```python
from build123d import *

# Parameters (mm, degrees)
SKETCH1_W            = 150
SKETCH1_H            = 150
BOSS_EXTRUDE2_DEPTH  = 3
SKETCH7_R            = 3
BOSS_EXTRUDE3_DEPTH  = 13
SKETCH13_W           = 15.146104274
SKETCH13_H           = 8
BOSS_EXTRUDE4_DEPTH  = 55
SKETCH14_W           = 100
SKETCH14_H           = 100
BOSS_EXTRUDE5_DEPTH  = 3
SKETCH15_R           = 3.001760758
SKETCH15_R_2         = 3.00141088
SKETCH15_R_3         = 3.000339641
SKETCH15_R_4         = 2.9990493
BOSS_EXTRUDE22_DEPTH = 15
SKETCH20_R           = 3
BOSS_EXTRUDE8_DEPTH  = 22.7
SKETCH23_W           = 52.466562125
SKETCH23_H           = 3
SKETCH23_W_2         = 9
BOSS_EXTRUDE9_DEPTH  = 5
BOSS_EXTRUDE10_DEPTH = 52.47
BOSS_EXTRUDE11_START = -74
BOSS_EXTRUDE11_DEPTH = 9
SKETCH25_W           = 9.00183775
SKETCH25_H           = 11.837712984
BOSS_EXTRUDE12_DEPTH = 8
SKETCH26_W           = 9
SKETCH26_H           = 5
SKETCH26_W_2         = 52.466562125
BOSS_EXTRUDE13_DEPTH = 43
SKETCH27_R           = 1.4
SKETCH27_W           = 35.7
SKETCH27_H           = 2.6
SKETCH27_W_2         = 23
SKETCH27_H_2         = 33
BOSS_EXTRUDE14_DEPTH = 2.4
SKETCH29_W           = 21.53
SKETCH29_H           = 48.531461908
BOSS_EXTRUDE15_DEPTH = 3
BOSS_EXTRUDE16_DEPTH = 21.53
BOSS_EXTRUDE17_DEPTH = 9
BOSS_EXTRUDE18_START = -30.53
BOSS_EXTRUDE18_DEPTH = 52.47
CUT_EXTRUDE5_DEPTH   = 8
BOSS_EXTRUDE19_DEPTH = 21.53
SKETCH21_R           = 1.5
BOSS_EXTRUDE20_DEPTH = 3
SKETCH17_R           = 1.5
BOSS_EXTRUDE21_DEPTH = 3
SKETCH15_3_R         = 1.75230345
SKETCH15_3_R_2       = 1.749240596
SKETCH15_3_R_3       = 1.752045419
SKETCH15_3_R_4       = 1.747263247
BOSS_EXTRUDE23_DEPTH = 18
SKETCH27_3_R         = 1.4
BOSS_EXTRUDE24_DEPTH = 4.4


with BuildPart() as part:
    # Sketch1 → Boss-Extrude2 (new body)
    with BuildSketch(Plane.XY):
        with Locations((121.156017968, 146.961713176)):
            Rectangle(SKETCH1_W, SKETCH1_H)
    extrude(amount=BOSS_EXTRUDE2_DEPTH)

    # Sketch7 → Boss-Extrude3 (add)
    with BuildSketch(Plane.XY):
        with Locations(Location((100.23733205, 77.422228763, 0), (0, 0, 180))):
            Circle(SKETCH7_R)
        with Locations(Location((177.53733205, 77.422228763, 0), (0, 0, 180))):
            Circle(SKETCH7_R)
        with Locations(Location((177.53733205, 119.222228763, 0), (0, 0, 180))):
            Circle(SKETCH7_R)
        with Locations(Location((100.23733205, 119.222228763, 0), (0, 0, 180))):
            Circle(SKETCH7_R)
    extrude(amount=BOSS_EXTRUDE3_DEPTH)

    # Sketch13 → Boss-Extrude4 (add)
    with BuildSketch(Plane.XY.offset(3)):
        Polygon((196.156017968, 213.964413798), (196.156017968, 221.961713176), (99.253187126, 221.961713176), (99.253187126, 213.964413798), (107.253187126, 213.964413798), align=None)
        Polygon((107.253187126, 213.964413798), (99.253187126, 213.964413798), (99.253187126, 126.654100723), (107.253187126, 126.654100723), (107.253187126, 136.806372616), (107.253187126, 144.806372616), align=None)
        Polygon((196.156017968, 136.806372616), (196.156017968, 144.806372616), (107.253187126, 144.806372616), (107.253187126, 136.806372616), (181.009913694, 136.806372616), align=None)
        with Locations((188.582965831, 132.806372616)):
            Rectangle(SKETCH13_W, SKETCH13_H)
    extrude(amount=BOSS_EXTRUDE4_DEPTH)

    # Sketch14 → Boss-Extrude5 (add)
    with BuildSketch(Plane.XY.offset(58)):
        with Locations((146.156017968, 171.961713176)):
            Rectangle(SKETCH14_W, SKETCH14_H)
    extrude(amount=BOSS_EXTRUDE5_DEPTH)

    # Sketch15 → Boss-Extrude22 (add)
    with BuildSketch(Plane.XY.offset(61)):
        with Locations(Location((103.656017968, 214.961713176, 0), (0, 0, 180))):
            Circle(SKETCH15_R)
        with Locations(Location((103.656017968, 129.961713176, 0), (0, 0, 180))):
            Circle(SKETCH15_R_2)
        with Locations(Location((188.656017968, 129.961713176, 0), (0, 0, 180))):
            Circle(SKETCH15_R_3)
        with Locations(Location((188.656017968, 214.961713176, 0), (0, 0, 180))):
            Circle(SKETCH15_R_4)
    extrude(amount=BOSS_EXTRUDE22_DEPTH)

    # Sketch20 → Boss-Extrude8 (add)
    with BuildSketch(Plane.XY.offset(3)):
        with Locations(Location((92.052701123, 214.281671575, 0), (0, 0, 180))):
            Circle(SKETCH20_R)
        with Locations(Location((52.052701123, 214.281671575, 0), (0, 0, 180))):
            Circle(SKETCH20_R)
        with Locations(Location((52.052701123, 174.281671575, 0), (0, 0, 180))):
            Circle(SKETCH20_R)
        with Locations(Location((92.052701123, 174.281671575, 0), (0, 0, 180))):
            Circle(SKETCH20_R)
        with Locations(Location((92.005217403, 161.997286282, 0), (0, 0, 180))):
            Circle(SKETCH20_R)
        with Locations(Location((52.005217403, 161.997286282, 0), (0, 0, 180))):
            Circle(SKETCH20_R)
        with Locations(Location((92.005217403, 121.997286282, 0), (0, 0, 180))):
            Circle(SKETCH20_R)
        with Locations(Location((52.005217403, 121.997286282, 0), (0, 0, 180))):
            Circle(SKETCH20_R)
    extrude(amount=BOSS_EXTRUDE8_DEPTH)

    # Sketch23 → Boss-Extrude9 (add)
    with BuildSketch(Plane.XZ.offset(-121.961713176)):
        with Locations((169.922736906, 59.5)):
            Rectangle(SKETCH23_W, SKETCH23_H)
        with Locations((117.656017968, 59.5)):
            Rectangle(SKETCH23_W_2, SKETCH23_H)
    extrude(amount=BOSS_EXTRUDE9_DEPTH)

    # Sketch24 → Boss-Extrude10 (add)
    with BuildSketch(Plane(origin=(196.156017968, 0, 0), x_dir=(0, 0, -1), z_dir=(1, 0, 0))):
        with BuildLine():
            Line((-58, 116.961713176), (-58, 128.806372616))
            Line((-58, 128.806372616), (-46.155340559, 128.806372616))
            ThreePointArc((-46.155340559, 128.806372616), (-49.624560989, 120.430933605), (-58, 116.961713176))
        make_face()
    extrude(amount=-BOSS_EXTRUDE10_DEPTH)

    # Sketch24<2> → Boss-Extrude11 (add)
    with BuildSketch(Plane(origin=(196.156017968, 0, 0), x_dir=(0, 0, -1), z_dir=(1, 0, 0)).offset(BOSS_EXTRUDE11_START)):
        with BuildLine():
            ThreePointArc((-58, 116.961713176), (-49.624560989, 120.430933605), (-46.155340559, 128.806372616))
            Line((-46.155340559, 128.806372616), (-58, 128.806372616))
            Line((-58, 128.806372616), (-58, 116.961713176))
        make_face()
    extrude(amount=-BOSS_EXTRUDE11_DEPTH)

    # Sketch25 → Boss-Extrude12 (add)
    with BuildSketch(Plane.XZ.offset(-136.806372616)):
        with Locations((117.656936843, 52.081143508)):
            Rectangle(SKETCH25_W, SKETCH25_H)
    extrude(amount=BOSS_EXTRUDE12_DEPTH)

    # Sketch26 → Boss-Extrude13 (add)
    with BuildSketch(Plane.XY.offset(61)):
        with Locations((117.656017968, 119.461713176)):
            Rectangle(SKETCH26_W, SKETCH26_H)
        with Locations((169.922736906, 119.461713176)):
            Rectangle(SKETCH26_W_2, SKETCH26_H)
    extrude(amount=BOSS_EXTRUDE13_DEPTH)

    # Sketch27 → Boss-Extrude14 (add)
    with BuildSketch(Plane.XY.offset(104)):
        with BuildLine():
            Line((113.156017968, 221.961713176), (113.156017968, 116.961713176))
            Line((113.156017968, 116.961713176), (122.156017968, 116.961713176))
            Line((122.156017968, 116.961713176), (122.156017968, 121.961713176))
            Line((122.156017968, 121.961713176), (143.689455843, 121.961713176))
            Line((143.689455843, 121.961713176), (143.689455843, 116.961713176))
            Line((143.689455843, 116.961713176), (196.156017968, 116.961713176))
            Line((196.156017968, 116.961713176), (196.156017968, 121.961713176))
            add(Edge.make_bspline(
                [(196.156017968, 121.961713176), (183.802165041, 122.519707419), (184.728927285, 132.962052817)],
                knots=[0, 0, 0, 1, 1, 1], degree=2))
            Line((184.728927285, 132.962052817), (184.728927285, 221.961713176))
            Line((184.728927285, 221.961713176), (113.156017968, 221.961713176))
        make_face()
        with Locations((123.722051557, 137.797431656)):
            Circle(SKETCH27_R, mode=Mode.SUBTRACT)
        with Locations((146.156017968, 132.877431656)):
            Rectangle(SKETCH27_W, SKETCH27_H, mode=Mode.SUBTRACT)
        with Locations((167.722051557, 137.797431656)):
            Circle(SKETCH27_R, mode=Mode.SUBTRACT)
        with Locations((132.189455843, 178.297431656)):
            Rectangle(SKETCH27_W_2, SKETCH27_H_2, mode=Mode.SUBTRACT)
        with Locations((123.722051557, 213.87831574)):
            Circle(SKETCH27_R, mode=Mode.SUBTRACT)
        with Locations((167.722051557, 213.87831574)):
            Circle(SKETCH27_R, mode=Mode.SUBTRACT)
    extrude(amount=BOSS_EXTRUDE14_DEPTH)

    # Sketch29 → Boss-Extrude15 (add)
    with BuildSketch(Plane(origin=(0, 221.961713176, 0), x_dir=(1, 0, 0), z_dir=(0, 1, 0))):
        with Locations((132.921017968, -82.134269046)):
            Rectangle(SKETCH29_W, SKETCH29_H)
    extrude(amount=BOSS_EXTRUDE15_DEPTH)

    # Sketch30 → Boss-Extrude16 (add)
    with BuildSketch(Plane.ZY.offset(-122.156017968)):
        with BuildLine():
            Line((57.868538092, 224.961713176), (57.868538092, 221.961713176))
            Line((57.868538092, 221.961713176), (54.868538092, 221.961713176))
            ThreePointArc((54.868538092, 221.961713176), (55.747217748, 224.083033519), (57.868538092, 224.961713176))
        make_face()
    extrude(amount=-BOSS_EXTRUDE16_DEPTH)

    # Sketch31 → Boss-Extrude17 (add)
    with BuildSketch(Plane.ZY.offset(-113.156017968)):
        with BuildLine():
            Line((104, 121.961713176), (98.905674281, 121.961713176))
            ThreePointArc((98.905674281, 121.961713176), (100.397767738, 125.563945438), (104, 127.056038895))
            Line((104, 127.056038895), (104, 121.961713176))
        make_face()
    extrude(amount=-BOSS_EXTRUDE17_DEPTH)

    # Sketch31<3> → Boss-Extrude18 (add)
    with BuildSketch(Plane.ZY.offset(-113.156017968).offset(BOSS_EXTRUDE18_START)):
        with BuildLine():
            Line((104, 121.961713176), (98.905674281, 121.961713176))
            ThreePointArc((98.905674281, 121.961713176), (100.397767738, 125.563945438), (104, 127.056038895))
            Line((104, 127.056038895), (104, 121.961713176))
        make_face()
    extrude(amount=-BOSS_EXTRUDE18_DEPTH)

    # Sketch33 → Cut-Extrude5 (cut)
    with BuildSketch(Plane.XY.offset(104)):
        Polygon((196.156017968, 121.961713176), (189.528499082, 123.368575123), (186.307168563, 125.915180821), (185.797122977, 127.056038895), (196.156017968, 127.056038895), align=None)
    extrude(amount=-CUT_EXTRUDE5_DEPTH, mode=Mode.SUBTRACT)

    # Sketch32 → Boss-Extrude19 (add)
    with BuildSketch(Plane.ZY.offset(-122.156017968)):
        with BuildLine():
            Line((104, 221.961713176), (104, 216.871001578))
            ThreePointArc((104, 216.871001578), (100.400323308, 218.362036484), (98.909288402, 221.961713176))
            Line((98.909288402, 221.961713176), (104, 221.961713176))
        make_face()
    extrude(amount=-BOSS_EXTRUDE19_DEPTH)

    # Sketch21 → Boss-Extrude20 (add)
    with BuildSketch(Plane.XY.offset(25.7)):
        with Locations((52.005217403, 161.997286282)):
            Circle(SKETCH21_R)
        with Locations((92.005217403, 161.997286282)):
            Circle(SKETCH21_R)
        with Locations((92.005217403, 121.997286282)):
            Circle(SKETCH21_R)
        with Locations((52.005217403, 121.984897708)):
            Circle(SKETCH21_R)
        with Locations((52.052701123, 214.281671575)):
            Circle(SKETCH21_R)
        with Locations((92.052701123, 214.281671575)):
            Circle(SKETCH21_R)
        with Locations((92.052701123, 174.269283002)):
            Circle(SKETCH21_R)
        with Locations((52.052701123, 174.269283002)):
            Circle(SKETCH21_R)
    extrude(amount=BOSS_EXTRUDE20_DEPTH)

    # Sketch17 → Boss-Extrude21 (add)
    with BuildSketch(Plane.XY.offset(13)):
        with Locations((100.23733205, 119.222228763)):
            Circle(SKETCH17_R)
        with Locations((100.23733205, 77.422228763)):
            Circle(SKETCH17_R)
        with Locations((177.53733205, 77.422228763)):
            Circle(SKETCH17_R)
        with Locations((177.53733205, 119.222228763)):
            Circle(SKETCH17_R)
    extrude(amount=BOSS_EXTRUDE21_DEPTH)

    # Sketch15<3> → Boss-Extrude23 (add)
    with BuildSketch(Plane.XY.offset(61)):
        with Locations((103.656017968, 214.961713176)):
            Circle(SKETCH15_3_R)
        with Locations((103.656017968, 129.961713176)):
            Circle(SKETCH15_3_R_2)
        with Locations((188.656017968, 129.961713176)):
            Circle(SKETCH15_3_R_3)
        with Locations((188.656017968, 214.961713176)):
            Circle(SKETCH15_3_R_4)
    extrude(amount=BOSS_EXTRUDE23_DEPTH)

    # Sketch27<3> → Boss-Extrude24 (add)
    with BuildSketch(Plane.XY.offset(104)):
        with Locations((167.722051557, 137.797431656)):
            Circle(SKETCH27_3_R)
        with Locations((123.722051557, 137.797431656)):
            Circle(SKETCH27_3_R)
        with Locations((123.722051557, 213.87831574)):
            Circle(SKETCH27_3_R)
        with Locations((167.722051557, 213.87831574)):
            Circle(SKETCH27_3_R)
    extrude(amount=BOSS_EXTRUDE24_DEPTH)


solid = part.part
```
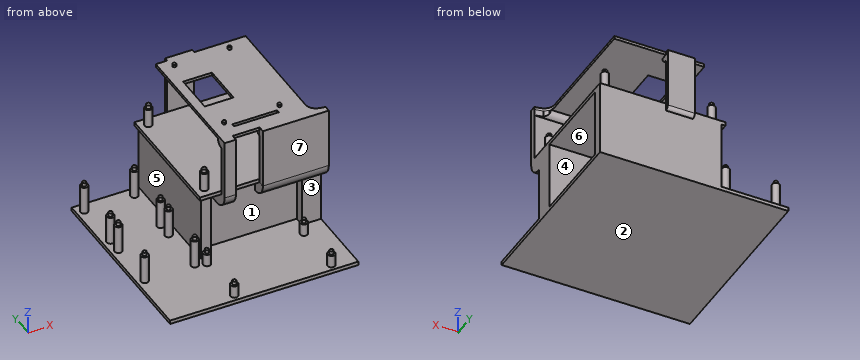
Here's how the part is built. I have some questions about the finished solid (model axes, mm). Face numbers are marked on the shaded views. A direction names the side the tool comes from. Round coordinates to 2 decimals unless told otherwise and drop trailing zeros. Write each loop counter-clockwise with the first axis right and the second up, starting at its lowest first coordinate (ties: lowest second). Pieces come first, ordered by that corner, then holes. Notation, with made-up numbers: M 40.25,-19 L 61.25,-19 A23 ccw 61.25,-10 Z; hole C 58.25,-24 d9. An arc over 180 degrees is marked long. Answer as CSV lines item,"result". Start each with the question number.
1. On a 3-axis mill with a long thin cutter (end or side, diameter ignored), from which of +Z, -Z, +X, -X, +Y, -Y can I reach the whole of each face in a straight line? I mean the marked faces 1, 2 and 3. Say none if no direction works.
2. Suppose I cut it at A-A on x = 130.5. Write out the boundary of the cut face in (y, z).
3. Thinking about a two-plate mould opening in Y: for the marked faces 4, 5, 6 and 7, which applies, released by +Y, released by -Y, zero draft, split by the parting line, or undercut?
4. Suppose I cut it at B-B on z = 92.5. Write out the boundary of the cut face in (x, y).
5. I need wall thicknesses on probe 1 along Z at (x, y) = (151, 191.5); probe 2 along X at (y, z) = (134, 51); probe 3 along Y at (x, z) = (170, 8). Which ranges of each line are inside material? Lowest first, please.
6. Suppose I cut it at C-C on y = 205.5. Write out the boundary of the cut face in (x, z).
7. Suppose I cut it at D-D on x = 157.5. Write out the boundary of the cut face in (y, z).
8. I'm going to push flat-ended pins straight in: pin 1 Ø1.5 at (x, z) = (128.5, 60) entering from -Y; pin 2 Ø19 at (x, z) = (175.5, 77) entering from +Y; pin 3 Ø5 at (x, z) = (97.5, 49.5) entering from +Y. Where does each tip first touch, or does it pass through?
Check result:
1,face 1,"none"
1,face 2,"-Z, +X, -X, +Y, -Y"
1,face 3,"+X, -Y"
2,outline,"M 71.96,0 L 221.96,0 L 221.96,54.87 A3 ccw 224.96,57.87 L 224.96,106.4 L 194.8,106.4 L 194.8,104 L 216.87,104 A5.09 ccw 221.96,98.91 L 221.96,61 L 121.96,61 L 121.96,58 L 136.81,58 L 136.81,3 L 71.96,3 Z; M 121.96,104 L 131.58,104 L 131.58,106.4 L 121.96,106.4 Z; M 134.18,104 L 161.8,104 L 161.8,106.4 L 134.18,106.4 Z; hole M 144.81,3 L 213.96,3 L 213.96,58 L 144.81,58 Z"
3,face 4,"undercut"
3,face 5,"zero draft"
3,face 6,"undercut"
3,face 7,"released by -Y"
4,outline,"M 113.16,116.96 L 122.16,116.96 L 122.16,121.96 L 113.16,121.96 Z; M 122.16,221.96 L 143.69,221.96 L 143.69,224.96 L 122.16,224.96 Z; M 143.69,116.96 L 196.16,116.96 L 196.16,121.96 L 143.69,121.96 Z"
5,probe 1,"z = 0 to 3, 58 to 61, 104 to 106.4"
5,probe 2,"x = 99.25 to 107.25, 113.16 to 122.16, 181.01 to 196.16"
5,probe 3,"y = 136.81 to 144.81, 213.96 to 221.96"
6,outline,"M 46.16,0 L 196.16,0 L 196.16,3 L 107.25,3 L 107.25,58 L 196.16,58 L 196.16,61 L 96.16,61 L 96.16,58 L 99.25,58 L 99.25,3 L 46.16,3 Z; M 113.16,104 L 184.73,104 L 184.73,106.4 L 113.16,106.4 Z"
7,outline,"M 71.96,0 L 221.96,0 L 221.96,61 L 121.96,61 L 121.96,98.91 A5.09 ccw 127.06,104 L 131.58,104 L 131.58,106.4 L 116.96,106.4 L 116.96,58 A11.84 ccw 128.81,46.16 L 128.81,58 L 136.81,58 L 136.81,3 L 71.96,3 Z; M 134.18,104 L 221.96,104 L 221.96,106.4 L 134.18,106.4 Z; hole M 144.81,3 L 213.96,3 L 213.96,58 L 144.81,58 Z"
8,pin 1,"stops at y = 121.96"
8,pin 2,"stops at y = 121.96"
8,pin 3,"stops at y = 221.96"
